Design review of the part built by this model. Coordinates are the model's own, in mm. Coordinates: 2 decimals unless noted, no trailing zeros. Loops run counter-clockwise (first coordinate to the right, second up) from the corner with the lowest first, then second, coordinate; pieces in that order, holes last. Notation, with made-up numbers: (42, -7.5) -> (84, -7.5) arc R15 ccw to (84, 7.5) -> close; hole circle Ø9 at (72, 11). An arc over 180 degrees is marked (long way). Use CSV: the item, a comma, the result in double quotes.
```python
from build123d import *

# Parameters (mm, degrees)
F0_W      = 31.75
F0_H      = 63.5
F1_DEPTH  = 3.175
F2_W      = 1.27
F2_H      = 3.175
F3_DEPTH  = 2.54
F4_W      = 1.27
F4_H      = 3.175
F5_DEPTH  = 2.54
F6_W      = 6.985
F6_H      = 3.175
F7_DEPTH  = 6.35
F9_DEPTH  = 25.4
F10_DEPTH = 25.4
F12_DEPTH = 9.55294
F11_W     = 6.985
F11_H     = 3.175
F13_DEPTH = 6.53796


with BuildPart() as f1:
    # F0 (on Top) → F1 (new body)
    with BuildSketch(Plane.XY):
        with Locations((15.875, 31.75)):
            Rectangle(F0_W, F0_H)
    extrude(amount=F1_DEPTH)

    # F2 (on face) → F3 (cut)
    with BuildSketch(Plane.YZ.offset(31.75)):
        with Locations((31.75, 1.5875)):
            Rectangle(F2_W, F2_H)
    extrude(amount=-F3_DEPTH, mode=Mode.SUBTRACT)

    # F4 (on face) → F5 (cut)
    with BuildSketch(Plane(origin=(0, 0, 0), x_dir=(0, -1, 0), z_dir=(-1, 0, 0))):
        with Locations((-31.75, 1.5875)):
            Rectangle(F4_W, F4_H)
    extrude(amount=-F5_DEPTH, mode=Mode.SUBTRACT)

    # F6 (on face) → F7 (join)
    with BuildSketch(Plane.XZ):
        with Locations((3.4925, 1.5875)):
            Rectangle(F6_W, F6_H)
        with Locations((28.2575, 1.5875)):
            Rectangle(F6_W, F6_H)
    extrude(amount=F7_DEPTH)

    # F8 (on face) → F9 (cut)
    with BuildSketch(Plane.XY.offset(3.175)):
        with BuildLine():
            ThreePointArc((5.29375, -4.35), (3.0318335149, -3.4130835149), (3.96875, -5.675))
            Line((3.96875, -5.675), (3.96875, -4.35))
            Line((3.96875, -4.35), (5.29375, -4.35))
        make_face()
        with BuildLine():
            Line((3.96875, -4.35), (3.96875, -5.675))
            ThreePointArc((3.96875, -5.675), (4.9056664851, -5.2869164851), (5.29375, -4.35))
            Line((5.29375, -4.35), (3.96875, -4.35))
        make_face()
        with BuildLine():
            ThreePointArc((29.10625, -4.35), (27.78125, -3.025), (26.45625, -4.35))
            Line((26.45625, -4.35), (27.78125, -4.35))
            Line((27.78125, -4.35), (27.78125, -5.675))
            ThreePointArc((27.78125, -5.675), (28.7181664851, -5.2869164851), (29.10625, -4.35))
        make_face()
        with BuildLine():
            Line((27.78125, -4.35), (26.45625, -4.35))
            ThreePointArc((26.45625, -4.35), (26.8443335149, -5.2869164851), (27.78125, -5.675))
            Line((27.78125, -5.675), (27.78125, -4.35))
        make_face()
    extrude(amount=-F9_DEPTH, mode=Mode.SUBTRACT)

    # F8 (on face) → F10 (cut)
    with BuildSketch(Plane.XY.offset(3.175)):
        with BuildLine():
            ThreePointArc((3.96875, 62.82602), (3.0318335149, 60.5641035149), (5.29375, 61.50102))
            ThreePointArc((5.29375, 61.50102), (4.9056664851, 62.4379364851), (3.96875, 62.82602))
        make_face()
        with BuildLine():
            ThreePointArc((27.78125, 62.82602), (26.8443335149, 62.4379364851), (26.45625, 61.50102))
            ThreePointArc((26.45625, 61.50102), (27.78125, 60.17602), (29.10625, 61.50102))
            ThreePointArc((29.10625, 61.50102), (28.7181664851, 62.4379364851), (27.78125, 62.82602))
        make_face()
    extrude(amount=-F10_DEPTH, mode=Mode.SUBTRACT)

    # F12 (add): faces of the model
    f12_faces = [f1.faces().sort_by_distance(p)[0] for p in [
        (28.2575, -6.35, 1.5875),
        (3.4925, -6.35, 1.5875),
    ]]
    extrude(f12_faces, amount=F12_DEPTH)

    # F11 (on face) → F13 (join)
    with BuildSketch(Plane(origin=(0, 63.5, 0), x_dir=(-1, 0, 0), z_dir=(0, 1, 0))):
        with Locations((-28.2575, 1.5875)):
            Rectangle(F11_W, F11_H)
        with Locations((-3.4925, 1.5875)):
            Rectangle(F11_W, F11_H)
    extrude(amount=F13_DEPTH)


solid = f1.part
```
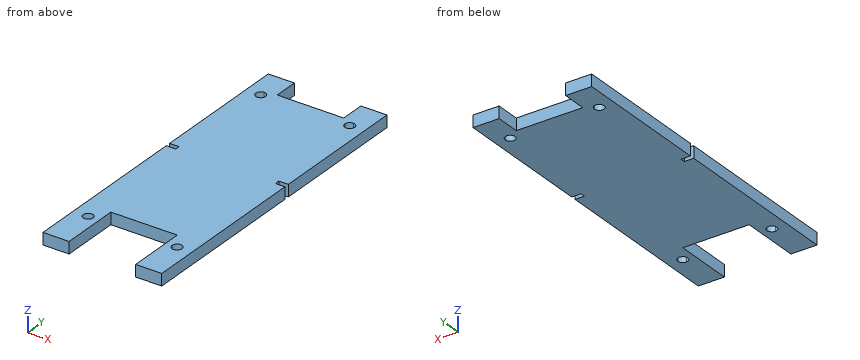
Item 1: Clearance check with flat-ended pins moving along their axes: pin 1 (1 mm diameter, centred on y = 31.5, z = 1, fed in from +X); pin 2 (1 mm diameter, centred on x = 17, z = 1.5, fed in from +Y); pin 3 (0.6 mm diameter, centred on y = 32, z = 1.5, fed in from -X). State where each tip first meets the part, or that it passes through.
Checked values:
pin 1,"x = 31.75"
pin 2,"y = 63.5"
pin 3,"x = 2.54"
Item 2: Add section A-A (y = -7). Give the boundary of the cut face in (x, z) (3 decimals), then the cut area to 3 significant figures.
Checked values:
outline,"(0, 0) -> (6.985, 0) -> (6.985, 3.175) -> (0, 3.175) -> close; (24.765, 0) -> (31.75, 0) -> (31.75, 3.175) -> (24.765, 3.175) -> close"
area,"44.4 mm^2"
Item 3: Add section C-C (x = 17.5). Give the boundary of the cut face in (y, z) (3 decimals).
Checked values:
outline,"(0, 0) -> (63.5, 0) -> (63.5, 3.175) -> (0, 3.175) -> close"
Item 4: Add section B-B (z = 1.3). Give the boundary of the cut face in (x, y) (3 decimals).
Checked values:
outline,"(0, -15.903) -> (6.985, -15.903) -> (6.985, 0) -> (24.765, 0) -> (24.765, -15.903) -> (31.75, -15.903) -> (31.75, 31.115) -> (29.21, 31.115) -> (29.21, 32.385) -> (31.75, 32.385) -> (31.75, 70.038) -> (24.765, 70.038) -> (24.765, 63.5) -> (6.985, 63.5) -> (6.985, 70.038) -> (0, 70.038) -> (0, 32.385) -> (2.54, 32.385) -> (2.54, 31.115) -> (0, 31.115) -> close; hole circle Ø2.65 at (3.969, -4.35); hole circle Ø2.65 at (3.969, 61.501); hole circle Ø2.65 at (27.781, -4.35); hole circle Ø2.65 at (27.781, 61.501)"
Item 5: To check wall thickness, follow line 1 along X through (y, z) = (-4.35, 2.3) (3 decimals); line 2 along X through (y, z) = (-8.5, 2.65) (3 decimals); line 3 along Y through (x, z) = (1, 2.5) (3 decimals). State the ranges of each line that lie inside material, in increasing order.
Checked values:
line 1,"0 to 2.644, 5.294 to 6.985, 24.765 to 26.456, 29.106 to 31.75"
line 2,"0 to 6.985, 24.765 to 31.75"
line 3,"-15.903 to 31.115, 32.385 to 70.038"
